Can you work these out from the model? Positions are in its coordinate system, mm. Face numbers are marked on the shaded views. A direction names the side the tool comes from. Give positions to 0.01 mm unless a question says otherwise; leave off trailing zeros. Loops run counter-clockwise (first coordinate to the right, second up) from the corner with the lowest first, then second, coordinate; pieces in that order, holes last. Notation, with made-up numbers: (-23.5, 41.5) - (-6.5, 41.5) arc R28 ccw to (-6.5, 59.5) - close; hole circle Ø7 at (37, 50.5). An arc over 180 degrees is marked (long way). Answer as a JSON object with one key per item and string values. Group by question number.
Item 1: Thinking about a two-plate mould opening in Y: for the marked faces 1, 2 and 3, which applies, pulls with the +Y half, pulls with the -Y half, needs draft (parallel to the pull), parting line crosses it, or undercut?
Item 2: Please list where these lines run through material, in increasing order: L1, parallel to X at y = 3, z = 19; L2, parallel to X at y = 12, z = 14; L3, parallel to Z at x = 90, y = 13.97.
Item 3: Suppose I cut it at D-D on y = 33.5. Write out the boundary of the cut face in (x, z) (1 decimal).
Item 4: Will these pins go through, and if not, where does the flat tip stop? pin 1 (0.5 mm diameter, centred on x = 24.5, z = 12.5, fed in from +Y) (3 decimals); pin 2 (0.5 mm diameter, centred on x = 3.5, z = 25, fed in from +Y) (3 decimals); pin 3 (0.5 mm diameter, centred on x = 14, z = 26.5, fed in from +Y) (3 decimals); pin 4 (2 mm diameter, centred on y = 14.5, z = 19.5, fed in from +X).
Item 5: Suppose I cut it at B-B on y = 13.97. Count the separate pieces of the cut face and the enclosed holes in it, and give its area (3 significant figures).
Item 6: Which directions (+Z, -Z, +X, -X, +Y, -Y) give clear straight access to the entire face, cutting with the end or side of a thin tool? Please do the marked faces 4, 5, 6 and 7.
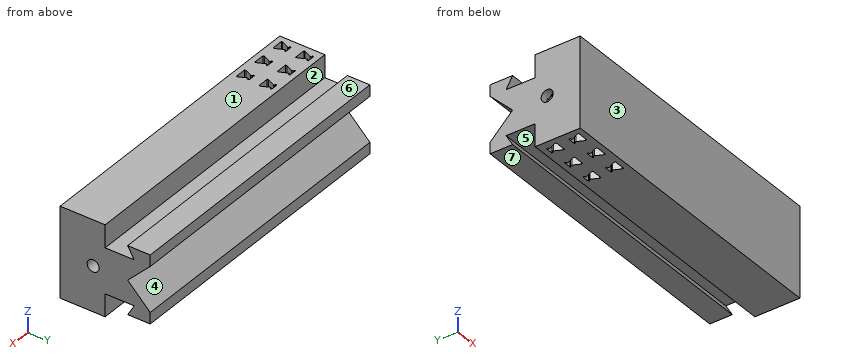
from build123d import *

# Parameters (mm, degrees)
BOSS_EXTRUDE2_DEPTH  = 19.05
BOSS_EXTRUDE1_DEPTH  = 127
SKETCH6_R            = 2.54
CUT_EXTRUDE2_DEPTH   = 128
CUT_EXTRUDE3_DEPTH   = 128
CUT_EXTRUDE4_DEPTH   = 39.1
LPATTERN1_COUNT      = 3
LPATTERN1_PITCH      = 10.583333333
LPATTERN1_COUNT_DIR2 = 2
LPATTERN1_PITCH_DIR2 = 9.525


with BuildPart() as part:
    # Base → Boss-Extrude2 (new body)
    with BuildSketch(Plane(origin=(0, 0, 0), x_dir=(1, 0, 0), z_dir=(0, 1, 0))):
        Polygon((0, 0), (63.5, 0), (122.112570575, 0), (127, 0), (127, -38.1), (31.75, -38.1), (0, -38.1), align=None)
    extrude(amount=BOSS_EXTRUDE2_DEPTH)

    # Sketch3 → Boss-Extrude1 (add)
    with BuildSketch(Plane(origin=(127, 0, 0), x_dir=(0, 0, -1), z_dir=(1, 0, 0))):
        Polygon((-38.1, 38.1), (-28.575, 38.1), (-19.05, 28.575), (-9.525, 38.1), (0, 38.1), (0, 0), (-38.1, 0), align=None)
    extrude(amount=-BOSS_EXTRUDE1_DEPTH)

    # Sketch6 → Cut-Extrude2 (cut, through all)
    with BuildSketch(Plane(origin=(127, 0, 0), x_dir=(0, 0, -1), z_dir=(1, 0, 0))):
        with Locations((-19.05, 13.97)):
            Circle(SKETCH6_R)
    extrude(amount=-CUT_EXTRUDE2_DEPTH, mode=Mode.SUBTRACT)

    # Sketch8 → Cut-Extrude3 (cut, through all)
    with BuildSketch(Plane(origin=(127, 0, 0), x_dir=(0, 0, -1), z_dir=(1, 0, 0))):
        Polygon((-4.7625, 28.575), (-4.7625, 38.1), (0, 38.1), (0, 19.05), (-9.525, 19.05), (-9.525, 31.324630657), align=None)
        Polygon((-28.575, 19.05), (-38.1, 19.05), (-38.1, 38.1), (-33.3375, 38.1), (-33.3375, 28.575), (-28.575, 31.324630657), align=None)
    extrude(amount=-CUT_EXTRUDE3_DEPTH, mode=Mode.SUBTRACT)

    # Sketch9 → Cut-Extrude4 (cut, through all)
    with BuildSketch(Plane.XY.offset(38.1)):
        Polygon((3.175, 16.66875), (6.35, 16.66875), (6.35, 16.0734375), (5.7546875, 16.0734375), (5.7546875, 15.478125), (7.14375, 12.5015625), (7.14375, 11.90625), (2.38125, 11.90625), (2.38125, 12.5015625), (3.7703125, 15.478125), (3.7703125, 16.0734375), (3.175, 16.0734375), align=None)
    cut_extrude4 = extrude(amount=-CUT_EXTRUDE4_DEPTH, mode=Mode.SUBTRACT)

    # LPattern1: Cut-Extrude4 3 × 2
    with Locations(*[(i * LPATTERN1_PITCH, -j * LPATTERN1_PITCH_DIR2, 0) for i in range(LPATTERN1_COUNT) for j in range(LPATTERN1_COUNT_DIR2) if (i, j) != (0, 0)]):
        add(cut_extrude4, mode=Mode.SUBTRACT)


solid = part.part
Worked out:
{
 "1": {"face 1": "needs draft", "face 2": "undercut", "face 3": "pulls with the -Y half"},
 "2": {"L1": "x = 0 to 2.39, 7.13 to 12.98, 17.72 to 23.56, 28.3 to 127", "L2": "x = 0 to 2.38, 7.14 to 12.96, 17.73 to 23.55, 28.31 to 127", "L3": "z = 0 to 16.51, 21.59 to 38.1"},
 "3": {"outline": "(0, 4.8) - (127, 4.8) - (127, 14.1) - (0, 14.1) - close; (0, 24) - (127, 24) - (127, 33.3) - (0, 33.3) - close"},
 "4": {"pin 1": "stops at y = 35.375", "pin 2": "stops at y = 34.775", "pin 3": "stops at y = 36.275", "pin 4": "passes through"},
 "5": {"separate pieces": "8", "enclosed holes": "0", "area": "3,860 mm2"},
 "6": {"face 4": "+X, -X, +Y", "face 5": "+X, -X", "face 6": "+Z, +X, -X, +Y", "face 7": "-Z, +X, -X, +Y"}
}
